CAD build for the part. Positions are in the model's coordinates, mm. A direction names the side the tool comes from. Coordinates: 2 decimals unless noted, no trailing zeros. Order: outer loops, then holes, each group sorted by start corner. A loop starts at its lowest first (then second) coordinate and runs counter-clockwise, first axis right, second up. Notation, with made-up numbers: (-18.75, 60) - (11.25, 60) arc R4 cw to (11.25, 66) - close; hole circle Ø7 at (9, 42). An arc over 180 degrees is marked (long way). Use one line per item in the form item = value.
Autodesk Inventor part; units mm, degrees
ref_plane "YZ Plane" through (0, 0, 0) normal (1, 0, 0) x (0, 1, 0)
ref_plane "XY Plane" through (0, 0, 0) normal (0, 0, 1) x (1, 0, 0)
sketch "Szkic1" plane through (0, 0, 0) normal (0, 0, 1) x (1, 0, 0)
  circle A0 centre (0, 0) radius 4.5
  dimension "d0" = 9
extrude "Wyciągnięcie proste1" add sketch "Szkic1" along normal blind 20
sketch "Szkic2" plane through (0, 0, 0) normal (0, 0, -1) x (-1, 0, 0)
  circle A0 centre (0, 0) radius 3
  dimension "d3" = 6
extrude "Wyciągnięcie proste2" cut sketch "Szkic2" against normal blind 17
sketch "Szkic3" plane through (0, 0, 20) normal (0, 0, 1) x (1, 0, 0)
  circle A0 centre (0, 0) radius 2.75
  line L0 (-2.3049, 1.5) -> (2.3049, 1.5)
  line L1 (-2.3049, -1.5) -> (2.3049, -1.5)
  dimension "d6" = 5.5
  dimension "d7" = 1.5
  dimension "d8" = 1.5
extrude "Wyciągnięcie proste3" add sketch "Szkic3" along normal blind 7 contours A0 L1 L0
ref_plane "Płaszczyzna konstrukcyjna1" through (0, 5, 0) normal (0, 1, 0) x (-1, 0, 0)
sketch "Szkic6" plane through (0, 5, 0) normal (0, 1, 0) x (-1, 0, 0)
  line L0 (-2.3049, 20) -> (-2.3049, 27)
  point P0 (0, 0)
  point P1 (-0.5435, 3.9629)
  point P2 (-0.5435, 13.9629)
  dimension "d12" = 10
  dimension "d13" = 4
  dimension "d14" = 1.7614
  dimension "d15" = 1.7614
hole "Otwór1" at (0.5435, 5, 3.9629) at (0.5435, 5, 13.9629) direction (0, -1, 0) diameter 3 end through all
properties part number "Ośka"
Item 1: Cut at A-A, the plane x = 0. Write the cut outline in (y, z), plus the area to 3 significant figures.
Derived:
outline = (-4.5, 0) - (-3, 0) - (-3, 2.56) - (-4.5, 2.56) - close; (-4.5, 5.36) - (-3, 5.36) - (-3, 12.56) - (-4.5, 12.56) - close; (-4.5, 15.36) - (-3, 15.36) - (-3, 17) - (3, 17) - (3, 15.36) - (4.5, 15.36) - (4.5, 20) - (1.5, 20) - (1.5, 27) - (-1.5, 27) - (-1.5, 20) - (-4.5, 20) - close; (3, 0) - (4.5, 0) - (4.5, 2.56) - (3, 2.56) - close; (3, 5.36) - (4.5, 5.36) - (4.5, 12.56) - (3, 12.56) - close
area = 82.2 mm²
Item 2: Cut at B-B, the plane y = 0. Write the cut outline in (x, z).
Derived:
outline = (-4.5, 0) - (-3, 0) - (-3, 17) - (3, 17) - (3, 0) - (4.5, 0) - (4.5, 20) - (2.75, 20) - (2.75, 27) - (-2.75, 27) - (-2.75, 20) - (-4.5, 20) - close
Item 3: Drill centre lines: line 1 (Z direction, x = 0.5, y = -3.25); line 2 (Z direction, x = -2.5, y = -3.5); line 3 (Z direction, x = -1.5, y = 0). Where is each one in solid material? Low to high. Write a range as [from, to].
Derived:
line_1 = [0, 2.46], [5.46, 12.46], [15.46, 20]
line_2 = [0, 20]
line_3 = [17, 27]
Item 4: Cut at D-D, the plane z = 10. Write the cut outline in (x, y).
Derived:
outline = circle Ø9 at (0, 0); hole circle Ø6 at (0, 0)
Item 5: Drop flat-ended pins along their axis: pin 1 (1.5 mm diameter, centred on x = -1.5, z = 9.5, fed in from +Y); pin 2 (1.4 mm diameter, centred on x = 1, z = 23, fed in from +Y); pin 3 (2 mm diameter, centred on x = 2.5, z = 18.5, fed in from +Y). Give the stop position or say it passes through.
Derived:
pin_1 = 4.44
pin_2 = 1.5
pin_3 = 4.24
Item 6: Cut at C-C, the plane z = 2.75. Write the cut outline in (x, y), plus the area to 3 significant figures.
Derived:
outline = (-0.34, -4.49) - (-0.34, -2.98) arc R3 cw to (-0.34, 2.98) - (-0.34, 4.49) arc R4.5 ccw to start; (1.43, -4.27) arc R4.5 ccw to (1.43, 4.27) - (1.43, 2.64) arc R3 cw to (1.43, -2.64) - close
area = 29.9 mm²
Item 7: 3-axis set-ups, long thin cutter, end or side, ignore diameter. For faces 5 (the face through (0, -1.5, 23)), 6 (the face through (-2.77, -1.15, 8.38)), 7 (the face through (0, 1.5, 23)): which of +Z, -Z, +X, -X, +Y, -Y reach the whole face in a straight line?
Derived:
face_5 = +Z, +X, -X, -Y
face_6 = -Z
face_7 = +Z, +X, -X, +Y
Item 8: Two-plate mould, pull along X, no slides. Class faces 1 (the face through (-2.75, -0.02, 23.45)), 2 (the face through (0.478, -3.62, 2.464)), 3 (the face through (1, -3, 0)), 4 (the face through (-0.98, 4.39, 9.86)): +X half, -X half, draft (parallel to the pull), parting line (faces both ways), or undercut.
Derived:
face_1 = -X half
face_2 = undercut
face_3 = draft
face_4 = parting line
